Part model, mm, in its own coordinate system. Coordinates: 2 decimals unless noted, no trailing zeros. Order: outer loops, then holes, each group sorted by start corner. A loop starts at its lowest first (then second) coordinate and runs counter-clockwise, first axis right, second up.
from build123d import *

# Parameters (mm, degrees)
SKETCH1_W           = 34
SKETCH1_H           = 14
BOSS_EXTRUDE1_DEPTH = 2
SKETCH3_R           = 1.5
CUT_EXTRUDE1_DEPTH  = 2
SKETCH4_R           = 1.5
CUT_EXTRUDE2_DEPTH  = 2


with BuildPart() as part:
    # Sketch1 → Boss-Extrude1 (new body)
    with BuildSketch(Plane(origin=(0.099311048, 0, 0), x_dir=(1, 0, 0), z_dir=(0, 0, 1))):
        with Locations((-20.155081556, 54.173525721)):
            Rectangle(SKETCH1_W, SKETCH1_H)
    extrude(amount=BOSS_EXTRUDE1_DEPTH)

    # Sketch3 → Cut-Extrude1 (cut)
    with BuildSketch(Plane(origin=(0.099311048, 0, 2), x_dir=(1, 0, 0), z_dir=(0, 0, 1))):
        with Locations((-25.558678377, 54.197225708)):
            Circle(SKETCH3_R)
    extrude(amount=-CUT_EXTRUDE1_DEPTH, mode=Mode.SUBTRACT)

    # Sketch4 → Cut-Extrude2 (cut)
    with BuildSketch(Plane(origin=(0.099311048, 0, 2), x_dir=(1, 0, 0), z_dir=(0, 0, 1))):
        with Locations((-19.918081695, 54.24462568)):
            Circle(SKETCH4_R)
        with Locations((-14.846284679, 54.24462568)):
            Circle(SKETCH4_R)
    extrude(amount=-CUT_EXTRUDE2_DEPTH, mode=Mode.SUBTRACT)


solid = part.part
Q1. Pin check, flat tip, straight feed: pin 1 Ø3.5 at (x, y) = (-19.82, 54.24) entering from +Z. Stop position of the tip, or through.
Results list:
pin 1: stops at z = 2
Q2. Cut at B-B on y = 53.25. Write the cut outline in (x, z).
Results list:
outline: (-37.06, 0) - (-26.62, 0) - (-26.62, 2) - (-37.06, 2) - close; (-24.3, 0) - (-20.94, 0) - (-20.94, 2) - (-24.3, 2) - close; (-18.7, 0) - (-15.87, 0) - (-15.87, 2) - (-18.7, 2) - close; (-13.62, 0) - (-3.06, 0) - (-3.06, 2) - (-13.62, 2) - close
Q3. Cut at A-A on z = 0.5. Write the cut outline in (x, y).
Results list:
outline: (-37.06, 47.17) - (-3.06, 47.17) - (-3.06, 61.17) - (-37.06, 61.17) - close; hole circle Ø3 at (-25.46, 54.2); hole circle Ø3 at (-19.82, 54.24); hole circle Ø3 at (-14.75, 54.24)
Q4. Wall check: line 1 along X through (y, z) = (54.25, 1.9); line 2 along X through (y, z) = (55.25, 1.7); line 3 along Y through (x, z) = (-16, 1.2). Give the ranges that are in metal, low to high.
Results list:
line 1: x = -37.06 to -26.96, -23.96 to -21.32, -18.32 to -16.25, -13.25 to -3.06
line 2: x = -37.06 to -26.53, -24.39 to -20.93, -18.71 to -15.86, -13.63 to -3.06
line 3: y = 47.17 to 53.42, 55.07 to 61.17
Q5. Mould opens along X. For faces 1 (the face through (-14.942, 55.732, 1.014)), 2 (the face through (-20, 61.174, 1)), 3 (the face through (-37.056, 54, 1)), 4 (the face through (-3.056, 54, 1)) say: pulls with the +X half, pulls with the -X half, needs draft (parallel to the pull), parting line crosses it, or undercut.
Results list:
face 1: undercut
face 2: needs draft
face 3: pulls with the -X half
face 4: pulls with the +X half
Q6. Cut at C-C on x = -14. Write the cut outline in (y, z).
Results list:
outline: (47.17, 0) - (52.94, 0) - (52.94, 2) - (47.17, 2) - close; (55.55, 0) - (61.17, 0) - (61.17, 2) - (55.55, 2) - close
